Input: part model. Units: mm. Frame: model coordinates. Face numbers are marked on the shaded views. A direction names the side the tool comes from. Coordinates: 2 decimals unless noted, no trailing zeros. Order: outer loops, then holes, each group sorted by start corner. A loop starts at its lowest first (then second) coordinate and runs counter-clockwise, first axis right, second up. Notation, with made-up numbers: (27, 68) -> (75, 68) arc R16 cw to (75, 80) -> close; hole circle Ø1 at (63, -8). An arc over 180 degrees is marked (long way). Write each question's results on one line, items separated by ' | '.
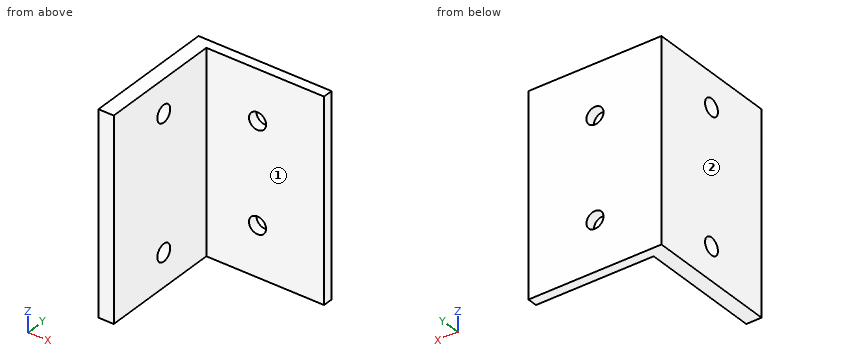
```python
from build123d import *

# Parameters (mm, degrees)
BOSS_EXTRUDE1_DEPTH                    = 76.2
F_0_257_DIAMETER_HOLE1_D               = 6.5278
F_0_257_DIAMETER_HOLE1_DEPTH           = 5.842
F_0_257_DIAMETER_HOLE1_ON_FACE_2_D     = 6.5278
F_0_257_DIAMETER_HOLE1_ON_FACE_2_DEPTH = 5.842


with BuildPart() as part:
    # Sketch1 → Boss-Extrude1 (new body)
    with BuildSketch(Plane.XY):
        Polygon((0, 0), (0, 50.8), (50.8, 50.8), (50.8, 46.99), (5.842, 46.99), (5.842, 0), align=None)
    extrude(amount=BOSS_EXTRUDE1_DEPTH)

    # F (0.257) Diameter Hole1
    with Locations(Plane(origin=(0, 25.4, 12.7), x_dir=(0, 0, -1), z_dir=(-1, 0, 0))):
        with Locations((0, 0), (-50.8, 0)):
            Hole(F_0_257_DIAMETER_HOLE1_D / 2, depth=F_0_257_DIAMETER_HOLE1_DEPTH)

    # F (0.257) Diameter Hole1 on face 2
    with Locations(Plane(origin=(25.4, 50.8, 19.05), x_dir=(0, 0, 1), z_dir=(0, 1, 0))):
        with Locations((0, 0), (38.1, 0)):
            Hole(F_0_257_DIAMETER_HOLE1_ON_FACE_2_D / 2, depth=F_0_257_DIAMETER_HOLE1_ON_FACE_2_DEPTH)


solid = part.part
```
(1) Cut plane D-D, the plane z = 19.05. Return loops of the section in (x, y).
Return value:
outline: (0, 0) -> (5.84, 0) -> (5.84, 46.99) -> (22.14, 46.99) -> (22.14, 50.8) -> (0, 50.8) -> close; (28.66, 46.99) -> (50.8, 46.99) -> (50.8, 50.8) -> (28.66, 50.8) -> close
(2) Line query: line 1 along Z through (x, y) = (4.3, 25.4); line 2 along X through (y, z) = (49.3, 57.15). Output: solid intervals per line, ascending. Write a range as from..to.
Return value:
line 1: 0..9.44, 15.96..60.24, 66.76..76.2 | line 2: 0..22.14, 28.66..50.8
(3) Pin query (flat end, axial travel): P1, Ø10.5, axis at x = 25.4, z = 57.15, coming from the -Y side; P2, Ø14, axis at y = 29.5, z = 21, coming from the +X side. Return the tip coordinate at first contact, or that it passes through.
Return value:
P1: y = 46.99 | P2: x = 5.84
(4) Reachability of the marked faces 1 and 2 from +Z, -Z, +X, -X, +Y, -Y: full face, straight path, thin tool, end or side. Return the list, or none.
Return value:
face 1: +Z, -Z, +X, -Y | face 2: +Z, -Z, -X, +Y, -Y
(5) Cut plane C-C, the plane y = 24. Return loops of the section in (x, z).
Return value:
outline: (0, 0) -> (5.84, 0) -> (5.84, 9.75) -> (0, 9.75) -> close; (0, 15.65) -> (5.84, 15.65) -> (5.84, 60.55) -> (0, 60.55) -> close; (0, 66.45) -> (5.84, 66.45) -> (5.84, 76.2) -> (0, 76.2) -> close
(6) Cut plane A-A, the plane x = 25.4. Return loops of the section in (y, z).
Return value:
outline: (46.99, 0) -> (50.8, 0) -> (50.8, 15.79) -> (46.99, 15.79) -> close; (46.99, 22.31) -> (50.8, 22.31) -> (50.8, 53.89) -> (46.99, 53.89) -> close; (46.99, 60.41) -> (50.8, 60.41) -> (50.8, 76.2) -> (46.99, 76.2) -> close
(7) Cut plane B-B, the plane z = 63.5. Return loops of the section in (x, y).
Return value:
outline: (0, 0) -> (5.84, 0) -> (5.84, 22.14) -> (0, 22.14) -> close; (0, 28.66) -> (5.84, 28.66) -> (5.84, 46.99) -> (50.8, 46.99) -> (50.8, 50.8) -> (0, 50.8) -> close
